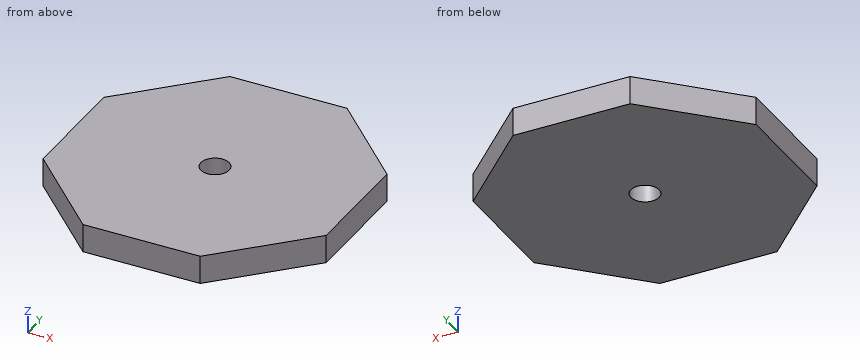
from build123d import *

# Parameters (mm, degrees)
F1_DEPTH = 6.35
F2_R     = 3.175
F3_DEPTH = 25.4


with BuildPart() as f1:
    # F0 (on Top) → F1 (new body)
    with BuildSketch(Plane.XY):
        Polygon((-31.75, 13.1512806053), (-31.75, -13.1512806053), (-13.1512806053, -31.75), (13.1512806053, -31.75), (31.75, -13.1512806053), (31.75, 13.1512806053), (13.1512806053, 31.75), (-13.1512806053, 31.75), align=None)
    extrude(amount=F1_DEPTH)

    # F2 (on face) → F3 (cut)
    with BuildSketch(Plane.XY.offset(6.35)):
        Circle(F2_R)
    extrude(amount=-F3_DEPTH, mode=Mode.SUBTRACT)


solid = f1.part
Read the model definition and answer for the solid it produces. Units are mm, in the model's axes. Round coordinates to 2 decimals unless told otherwise and drop trailing zeros. Order: outer loops, then holes, each group sorted by start corner. A loop starts at its lowest first (then second) coordinate and runs counter-clockwise, first axis right, second up.
1) The part is cut by section D-D on y = 14. Write down the section's boundary in (x, z).
2) The part is cut by section A-A on x = 0. Write down the section's boundary in (y, z) (3 decimals), plus the area to 3 significant figures.
3) Straight lines are drawn through the part: L1, parallel to Y at x = 0, z = 1.5 (3 decimals); L2, parallel to Y at x = 1.5, z = 4; L3, parallel to Y at x = 23, z = 4. For each, find the intervals that lie inside material, in ascending order.
4) A flat-ended cylindrical pin translates along its axis: pin 1 (5 mm diameter, centred on x = 0, y = 0, fed in from -Z). Find the tip coordinate at first contact, or state that the pin passes through.
5) The part is cut by section C-C on z = 3.5. Write down the section's boundary in (x, y) (3 decimals), plus the area to 3 significant figures.
Resolved:
1. outline: (-30.9, 0) - (30.9, 0) - (30.9, 6.35) - (-30.9, 6.35) - close
2. outline: (-31.75, 0) - (-3.175, 0) - (-3.175, 6.35) - (-31.75, 6.35) - close; (3.175, 0) - (31.75, 0) - (31.75, 6.35) - (3.175, 6.35) - close
2. area: 363 mm2
3. L1: y = -31.75 to -3.175, 3.175 to 31.75
3. L2: y = -31.75 to -2.8, 2.8 to 31.75
3. L3: y = -21.9 to 21.9
4. pin 1: passes through
5. outline: (-31.75, -13.151) - (-13.151, -31.75) - (13.151, -31.75) - (31.75, -13.151) - (31.75, 13.151) - (13.151, 31.75) - (-13.151, 31.75) - (-31.75, 13.151) - close; hole circle Ø6.35 at (0, 0)
5. area: 3,310 mm2
